Could you check a few things on this model? Use its own coordinates, in mm. Round coordinates to 2 decimals unless told otherwise and drop trailing zeros. Order: outer loops, then holes, each group sorted by start corner. A loop starts at its lowest first (then second) coordinate and runs counter-clockwise, first axis right, second up. Notation, with made-up numbers: (-21.75, 15.25) -> (37.25, 15.25) arc R24 cw to (37.25, 28.25) -> close; hole circle Ø7 at (-20.5, 85). An arc over 180 degrees is marked (long way). One line per question, with ' | ' between items.
```python
from build123d import *

# Parameters (mm, degrees)
F1_DEPTH = 0.6


with BuildPart() as f1:
    # F0 (on Front) → F1 (new body)
    with BuildSketch(Plane.XZ):
        Polygon((-9.3927199472, 0), (-9.1270949472, 1.7), (-9.0333449472, 2.3), (-9.640625, 2.3), (-10, 0), align=None)
        Polygon((-9.640625, 2.3), (-9.0333449472, 2.3), (-7.6189836648, 11.3519122078), (-7.5645949472, 11.7), (-7.5200572692, 11.9850411396), (-8.078125, 12.3), align=None)
        Polygon((-6.515625, 22.3), (-8.078125, 12.3), (-7.3980295932, 12.7660182659), (-6.0020949472, 21.7), (-5.9083449472, 22.3), align=None)
        Polygon((-5, 32), (-6.515625, 22.3), (-5.9083449472, 22.3), (-4.5716713254, 30.8547111795), (-4.4864699472, 31.4), (-4.287693299, 31.4), align=None)
        Polygon((5.8163040642, 22.8890616512), (6.515625, 22.3), (5, 32), (0, 32), (0, 31.4), (4.4864699472, 31.4), align=None)
        Polygon((0, 32), (-5, 32), (-4.287693299, 31.4), (0, 31.4), align=None)
        Polygon((7.4708449472, 12.3), (8.078125, 12.3), (6.515625, 22.3), (5.9670760935, 21.9241206637), (6.0020949472, 21.7), (6.0697327931, 21.2671177867), align=None)
        Polygon((7.5645949472, 11.7), (8.9746138009, 2.6758793363), (9.640625, 2.3), (8.078125, 12.3), (7.4708449472, 12.3), align=None)
        Polygon((9.0333449472, 2.3), (9.1270949472, 1.7), (9.3927199472, 0), (10, 0), (9.640625, 2.3), align=None)
        Polygon((0, 2.3), (0, 1.7), (9.1270949472, 1.7), (9.0333449472, 2.3), (8.4198732785, 2.3), align=None)
        Polygon((-9.1270949472, 1.7), (0, 1.7), (0, 2.3), (-9.0333449472, 2.3), align=None)
        Polygon((0, 7.7409171076), (0, 7.0519567004), (8.4198732785, 2.3), (9.0333449472, 2.3), (8.9746138009, 2.6758793363), align=None)
        Polygon((-7.6189836648, 11.3519122078), (0, 7.0519567004), (0, 7.7409171076), (-7.015, 11.7), (-7.5645949472, 11.7), align=None)
        Polygon((0, 12.3), (0, 11.7), (7.5645949472, 11.7), (7.4708449472, 12.3), align=None)
        Polygon((-7.015, 11.7), (0, 11.7), (0, 12.3), (-7.0166547269, 12.3), (-7.4708449472, 12.3), (-7.5200572692, 11.9850411396), align=None)
        Polygon((0, 17.8353319058), (0, 17.1079861084), (6.0697327931, 21.2671177867), (6.0020949472, 21.7), (5.64, 21.7), align=None)
        Polygon((-7.3980295932, 12.7660182659), (-7.4708449472, 12.3), (-7.0166547269, 12.3), (0, 17.1079861084), (0, 17.8353319058), align=None)
        Polygon((5.5842921721, 22.3), (5.9083449472, 22.3), (5.8163040642, 22.8890616512), (0, 27.7883310719), (0, 27.0038379653), align=None)
        Polygon((0, 27.7883310719), (-4.287693299, 31.4), (-4.4864699472, 31.4), (-4.5716713254, 30.8547111795), (0, 27.0038379653), align=None)
        Polygon((5.9670760935, 21.9241206637), (5.9083449472, 22.3), (5.5842921721, 22.3), (0, 22.3), (0, 21.7), (5.64, 21.7), align=None)
        Polygon((0, 22.3), (-5.9083449472, 22.3), (-6.0020949472, 21.7), (0, 21.7), align=None)
        Polygon((5.9083449472, 22.3), (6.515625, 22.3), (5.8163040642, 22.8890616512), align=None)
        Polygon((5.9670760935, 21.9241206637), (6.515625, 22.3), (5.9083449472, 22.3), align=None)
        Polygon((6.0020949472, 21.7), (5.9670760935, 21.9241206637), (5.64, 21.7), align=None)
        Polygon((8.9746138009, 2.6758793363), (9.0333449472, 2.3), (9.640625, 2.3), align=None)
        Polygon((-7.3980295932, 12.7660182659), (-8.078125, 12.3), (-7.4708449472, 12.3), align=None)
        Polygon((-7.4708449472, 12.3), (-8.078125, 12.3), (-7.5200572692, 11.9850411396), align=None)
        Polygon((-7.5645949472, 11.7), (-7.015, 11.7), (-7.5200572692, 11.9850411396), align=None)
    extrude(amount=F1_DEPTH)


solid = f1.part
```
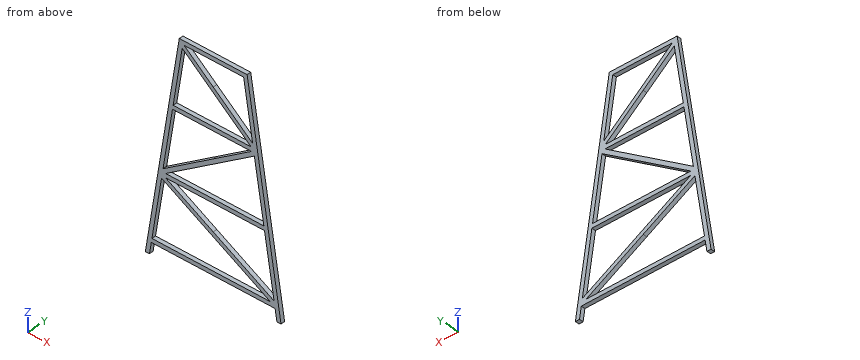
1. I want a section at B-B on y = -0.45. List the corners of the cut face in (x, z) for me (3 decimals).
From the geometry:
outline: (-10, 0) -> (-9.393, 0) -> (-9.127, 1.7) -> (9.127, 1.7) -> (9.393, 0) -> (10, 0) -> (5, 32) -> (-5, 32) -> close; hole (-9.033, 2.3) -> (8.42, 2.3) -> (-7.619, 11.352) -> close; hole (-7.398, 12.766) -> (5.64, 21.7) -> (-6.002, 21.7) -> close; hole (-7.017, 12.3) -> (7.471, 12.3) -> (6.07, 21.267) -> close; hole (-7.015, 11.7) -> (8.975, 2.676) -> (7.565, 11.7) -> close; hole (-5.908, 22.3) -> (5.584, 22.3) -> (-4.572, 30.855) -> close; hole (-4.288, 31.4) -> (5.816, 22.889) -> (4.486, 31.4) -> close
2. I'm going to push a flat-ended pin straight in: pin 1 (1 mm diameter, centred on x = -4.5, z = 23.5, fed in from -Y). Where does the tip first touch, or does it pass through?
From the geometry:
pin 1: passes through
3. I want a section at D-D on x = -5.5. List the corners of the cut face in (y, z) for me, and give its area (3 significant figures).
From the geometry:
outline: (-0.6, 1.7) -> (0, 1.7) -> (0, 2.3) -> (-0.6, 2.3) -> close; (-0.6, 10.16) -> (0, 10.16) -> (0, 10.84) -> (-0.6, 10.84) -> close; (-0.6, 11.7) -> (0, 11.7) -> (0, 12.3) -> (-0.6, 12.3) -> close; (-0.6, 13.34) -> (0, 13.34) -> (0, 14.07) -> (-0.6, 14.07) -> close; (-0.6, 21.7) -> (0, 21.7) -> (0, 22.3) -> (-0.6, 22.3) -> close; (-0.6, 24.91) -> (0, 24.91) -> (0, 28.8) -> (-0.6, 28.8) -> close | area: 4.26 mm²
4. I need wall thicknesses on probe 1 along X at (y, z) = (-0.15, 7); probe 2 along X at (y, z) = (-0.1, 28) (3 decimals); probe 3 along Z at (x, y) = (-4.5, -0.25). Which ranges of each line are inside material? Lowest first, please.
From the geometry:
probe 1: x = -8.91 to -8.3, 0.09 to 1.31, 8.3 to 8.91 | probe 2: x = -5.625 to -5.018, -1.183 to -0.251, 5.018 to 5.625 | probe 3: z = 1.7 to 2.3, 9.59 to 10.28, 11.7 to 12.3, 14.02 to 14.75, 21.7 to 22.3, 30.79 to 32
5. I want a section at C-C on z = 16.5. List the corners of the cut face in (x, y) for me, and give its area (3 significant figures).
From the geometry:
outline: (-7.42, -0.6) -> (-6.81, -0.6) -> (-6.81, 0) -> (-7.42, 0) -> close; (-1.95, -0.6) -> (-0.89, -0.6) -> (-0.89, 0) -> (-1.95, 0) -> close; (6.81, -0.6) -> (7.42, -0.6) -> (7.42, 0) -> (6.81, 0) -> close | area: 1.37 mm²
6. I want a section at A-A on x = 2.5. List the corners of the cut face in (y, z) for me.
From the geometry:
outline: (-0.6, 1.7) -> (0, 1.7) -> (0, 2.3) -> (-0.6, 2.3) -> close; (-0.6, 5.64) -> (0, 5.64) -> (0, 6.33) -> (-0.6, 6.33) -> close; (-0.6, 11.7) -> (0, 11.7) -> (0, 12.3) -> (-0.6, 12.3) -> close; (-0.6, 18.82) -> (0, 18.82) -> (0, 19.55) -> (-0.6, 19.55) -> close; (-0.6, 21.7) -> (0, 21.7) -> (0, 22.3) -> (-0.6, 22.3) -> close; (-0.6, 24.9) -> (0, 24.9) -> (0, 25.68) -> (-0.6, 25.68) -> close; (-0.6, 31.4) -> (0, 31.4) -> (0, 32) -> (-0.6, 32) -> close
